```python
from build123d import *

# Parameters (mm, degrees)
F0_W     = 5
F0_H     = 5
F1_DEPTH = 3
F2_W     = 5
F2_H     = 5
F3_DEPTH = 2
F4_SIZE  = 1.99999


# Not quite as in the source:
# - a fillet or chamfer is up to 0.001 mm smaller than in the source, because OpenCascade refuses the exact size


with BuildPart() as f1:
    # F0 (on Right) → F1 (new body)
    with BuildSketch(Plane.YZ):
        with Locations((40.6040474772, 32.0952650385)):
            Rectangle(F0_W, F0_H)
    extrude(amount=F1_DEPTH)

    # F2 (on face) → F3 (join)
    with BuildSketch(Plane(origin=(0, 0, 0), x_dir=(0, -1, 0), z_dir=(-1, 0, 0))):
        with Locations((-40.6040474772, 32.0952650385)):
            Rectangle(F2_W, F2_H)
        Polygon((-37.1040474772, 28.5952650385), (-37.1040474772, 35.5952650385), (-43.1040474772, 35.5952650385), (-43.1040474772, 34.5952650385), (-38.1040474772, 34.5952650385), (-38.1040474772, 29.5952650385), (-43.1040474772, 29.5952650385), (-43.1040474772, 28.5952650385), align=None)
        Polygon((-43.1040474772, 34.5952650385), (-43.1040474772, 35.5952650385), (-51.1040474772, 32.7952650385), (-51.1040474772, 31.3952650385), (-43.1040474772, 28.5952650385), (-43.1040474772, 29.5952650385), align=None)
        Polygon((-51.1040474772, 32.7952650385), (-43.1040474772, 35.5952650385), (-51.1040474772, 35.5952650385), align=None)
        Polygon((-51.1040474772, 32.7952650385), (-51.1040474772, 35.5952650385), (-53.1040474772, 35.5952650385), (-53.1040474772, 32.0952650385), align=None)
        Polygon((-51.1040474772, 31.3952650385), (-51.1040474772, 32.7952650385), (-53.1040474772, 32.0952650385), align=None)
    extrude(amount=F3_DEPTH)

    # F4 (size 2 in the source; OpenCascade refuses exactly that, so slightly less here)
    f4_edges = [f1.edges().sort_by_distance(p)[0] for p in [
        (-2, 37.104047, 32.095265),
    ]]
    chamfer(f4_edges, length=F4_SIZE)


solid = f1.part
```
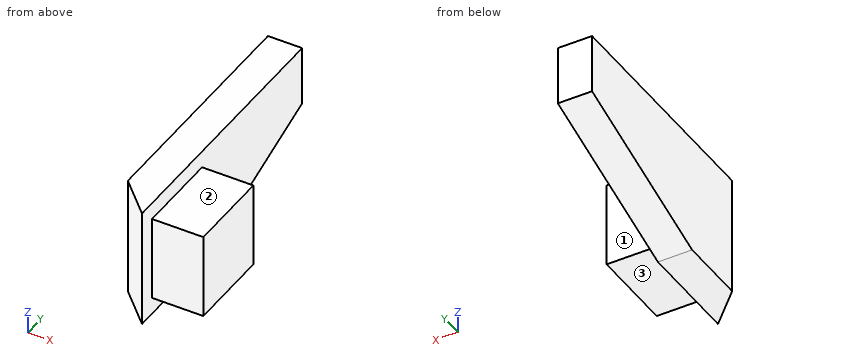
The listing builds one solid part. Answer for the finished solid, in the listing's coordinates (mm). Face numbers are marked on the shaded views. A direction names the side the tool comes from. Give positions to 0.01 mm unless a question says otherwise; leave off trailing zeros. Write each loop counter-clockwise with the first axis right and the second up, starting at its lowest first coordinate (ties: lowest second). Pieces come first, ordered by that corner, then holes. Notation, with made-up numbers: (12, 21) -> (35, 21) arc R11 cw to (35, 28) -> close; hole circle Ø2 at (-39, 66.5). An arc over 180 degrees is marked (long way). Write item = value, one per line. Start each with the question number.
1) Each of these flat-tipped pins is pushed along its axis until it touches: pin 1 (1.5 mm diameter, centred on x = 1, y = 41, fed in from -Z); pin 2 (2 mm diameter, centred on y = 47.5, z = 31, fed in from +X); pin 3 (1.5 mm diameter, centred on x = 1, z = 32.5, fed in from -Y). Where does it stop, or does it pass through?
2) Straight lines are drawn through the part: line 1 along X through (y, z) = (44.75, 30.75); line 2 along Y through (x, z) = (1.3, 33.25); line 3 along Z through (x, y) = (1.55, 42.75). For each, find the intervals that lie inside material, in ascending order.
3) The part is cut by section A-A, the plane y = 40.25. Determine the outline of the cut face in (x, z).
4) The part is cut by section C-C, the plane x = 0.4. Determine the outline of the cut face in (y, z).
5) Which of the six approach directions +Z, -Z, +X, -X, +Y, -Y give full straight-line access (tool end or side, diameter ignored) to the marked faces 1, 2 and 3?
Solutions:
q1.pin_1 = 29.6
q1.pin_2 = 0
q1.pin_3 = 38.1
q2.line_1 = -2 to 0
q2.line_2 = 38.1 to 43.1
q2.line_3 = 29.6 to 34.6
q3.outline = (-2, 28.6) -> (0, 28.6) -> (0, 29.6) -> (3, 29.6) -> (3, 34.6) -> (0, 34.6) -> (0, 35.6) -> (-2, 35.6) -> close
q4.outline = (38.1, 29.6) -> (43.1, 29.6) -> (43.1, 34.6) -> (38.1, 34.6) -> close
q5.face_1 = +Z, -Z, +X, +Y
q5.face_2 = +Z, +X, +Y, -Y
q5.face_3 = -Z, +X, +Y, -Y
